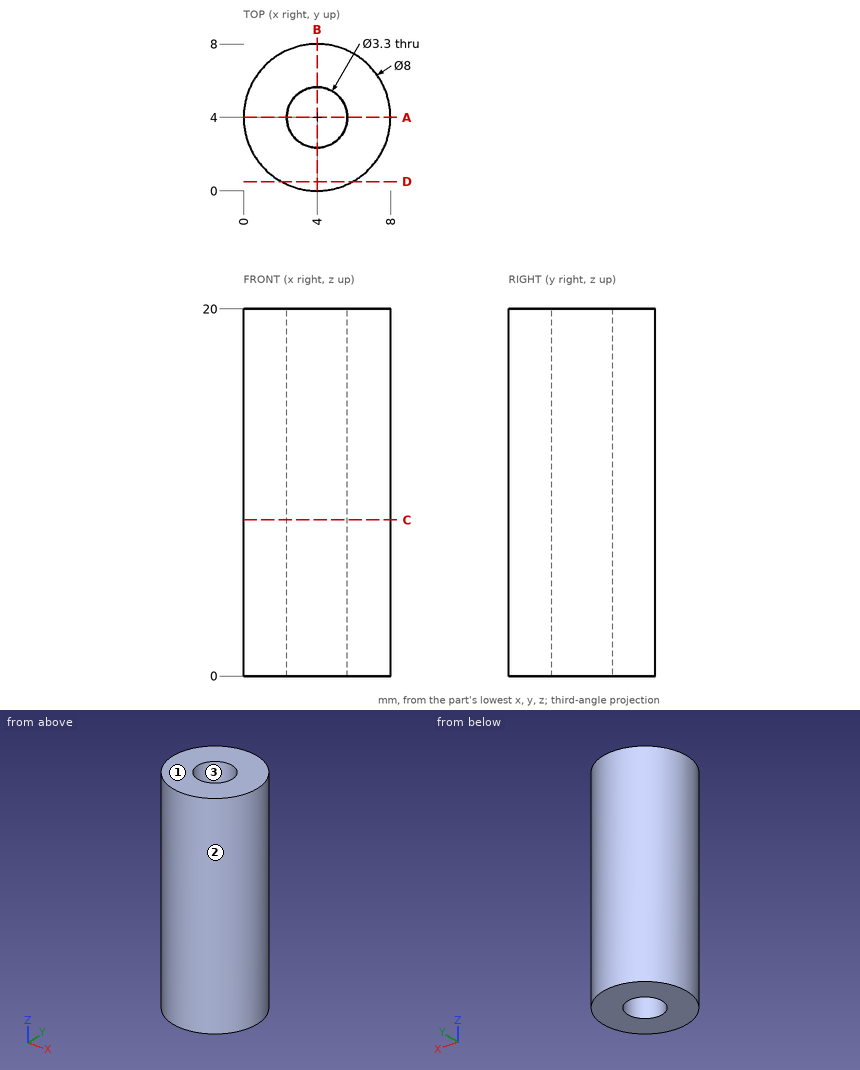
Check sheet for the drawn part. Datum: minimum x, y, z corner. Units: mm. Round coordinates to 2 decimals unless told otherwise and drop trailing zeros. Order: outer loops, then holes, each group sorted by start corner. A loop starts at its lowest first (then second) coordinate and runs counter-clockwise, first axis right, second up.
1) Section check D-D (y = 0.5). Record the boundary of the cut face in (x, z).
2) Mould release check, pull along X, two halves, no side actions. Record for the marked faces 1, 2 and 3: +X half, -X half, draft (parallel to the pull), parting line (faces both ways), or undercut.
3) Section check A-A (y = 4). Record the boundary of the cut face in (x, z).
4) Scan lines: line 1 (Y direction, x = 4, z = 4.75); line 2 (X direction, y = 3, z = 12.25); line 3 (X direction, y = 5.5, z = 16). Record each from-to range of solid material in increasing order.
5) Go/stop test with flat-tipped pins: pin 1 Ø1.5 at (x, z) = (6, 3) entering from -Y; pin 2 Ø3 at (x, y) = (4, 4) entering from +Z; pin 3 Ø3 at (y, z) = (1.5, 17.5) entering from +X. Record where each tip stops, or that it passes through.
6) Section check C-C (z = 8.5). Record the boundary of the cut face in (x, y), and give its area (3 significant figures).
Result:
1. outline: (2.06, 0) - (5.94, 0) - (5.94, 20) - (2.06, 20) - close
2. face 1: draft
2. face 2: parting line
2. face 3: undercut
3. outline: (0, 0) - (2.35, 0) - (2.35, 20) - (0, 20) - close; (5.65, 0) - (8, 0) - (8, 20) - (5.65, 20) - close
4. line 1: y = 0 to 2.35, 5.65 to 8
4. line 2: x = 0.13 to 2.69, 5.31 to 7.87
4. line 3: x = 0.29 to 3.31, 4.69 to 7.71
5. pin 1: stops at y = 0.2
5. pin 2: passes through
5. pin 3: stops at x = 7.87
6. outline: circle Ø8 at (4, 4); hole circle Ø3.3 at (4, 4)
6. area: 41.7 mm2
